Source: CAD feature listing. Evaluate the final solid. Frame: model axes, mm. A direction names the side the tool comes from. Round coordinates to 2 decimals unless told otherwise and drop trailing zeros. Order: outer loops, then holes, each group sorted by start corner. A loop starts at its lowest first (then second) coordinate and runs counter-clockwise, first axis right, second up. Notation, with made-up numbers: M 16.25,-26.5 L 46.25,-26.5 A30 ccw 46.25,-3.5 Z; hole C 10,81 d8. An arc over 180 degrees is marked long. Use one line per item in the form item = value. Start each with the question number.
Q1. Reachability of faces 1 (the flat face through (45, 10, 0.745)), 2 (the flat face through (45, -10, -0.745)), 3 (the cylindrical face through (4.7, 11.51, 3.62)) from +Z, -Z, +X, -X, +Y, -Y: full face, straight path, thin tool, end or side. Return the list, or none.
Q2. Section C-C (y = 0). Return the cut outline in (x, z) (3 decimals).
Q3. Pull-direction query (Y, two-part tool) for faces 4 (the cylindrical face through (50.978, 0.059, 3.174)), 5 (the cylindrical face through (36.13, 16.1, 5.07)), 6 (the flat face through (9.525, 11, -7)); classes: pulls with the +Y half, pulls with the -Y half, needs draft (parallel to the pull), parting line crosses it, or undercut.
Q4. Section A-A (x = 51). Return the cut outline in (y, z) (3 decimals), plus the area to 3 significant figures.
Q5. Material intervals for probe 1 along Z at (x, y) = (0.5, -0.5); probe 2 along Z at (x, y) = (51.5, 9), sorted ascending.
Q6. Section D-D (x = 16). Return the cut outline in (y, z).
Q7. Section B-B (z = 4.5). Return the cut outline in (x, y) (3 decimals).
Q8. Contact query for flat-ended pins moving along their axis: pin 1 (11 mm diameter, centred on x = 49.5, y = 7, fed in from -Z); pin 2 (6 mm diameter, centred on x = 5, z = -6, fed in from -Y); pin 3 (4 mm diameter, centred on x = 11, y = -2.5, fed in from -Z). Output: stop coordinate, or through.
from build123d import *

# Parameters (mm, degrees)
F0_R     = 12.065
F1_DEPTH = 9.525
F2_R     = 16.8783
F2_R_2   = 12.065
F3_DEPTH = 53.975
F4_R     = 12.7
F4_R_2   = 12.065
F5_DEPTH = 38.1
F6_R     = 3.175
F7_DEPTH = 25.4
F9_DEPTH = 38.1


with BuildPart() as f1:
    # F0 (on Right) → F1 (new body)
    with BuildSketch(Plane.YZ):
        Circle(F0_R)
    extrude(amount=F1_DEPTH)

    # F2 (on face) → F3 (join)
    with BuildSketch(Plane.YZ.offset(9.525)):
        Circle(F2_R)
        Circle(F2_R_2, mode=Mode.SUBTRACT)
        Circle(F2_R_2)
    extrude(amount=F3_DEPTH)

    # F4 (on face) → F5 (join)
    with BuildSketch(Plane(origin=(0, 0, 0), x_dir=(0, -1, 0), z_dir=(-1, 0, 0))):
        Circle(F4_R)
        Circle(F4_R_2, mode=Mode.SUBTRACT)
        Circle(F4_R_2)
    extrude(amount=F5_DEPTH)

    # F6 (on face) → F7 (cut)
    with BuildSketch(Plane.YZ.offset(63.5)):
        Circle(F6_R)
    extrude(amount=-F7_DEPTH, mode=Mode.SUBTRACT)

    # F8 (on face) → F9 (cut)
    with BuildSketch(Plane.YZ.offset(63.5)):
        with BuildLine():
            ThreePointArc((-16.8618667917, 0.7446201635), (-16.8783, 0), (-16.8618667917, -0.7446201635))
            Line((-16.8618667917, -0.7446201635), (-3.086448738, -0.7446201635))
            ThreePointArc((-3.086448738, -0.7446201635), (-3.175, 0), (-3.086448738, 0.7446201635))
            Line((-3.086448738, 0.7446201635), (-16.8618667917, 0.7446201635))
        make_face()
        with BuildLine():
            Line((3.086448738, -0.7446201635), (16.8618667917, -0.7446201635))
            ThreePointArc((16.8618667917, -0.7446201635), (16.8741911978, -0.3724007378), (16.8783, 0))
            ThreePointArc((16.8783, 0), (16.8741911978, 0.3724007378), (16.8618667917, 0.7446201635))
            Line((16.8618667917, 0.7446201635), (3.086448738, 0.7446201635))
            ThreePointArc((3.086448738, 0.7446201635), (3.1527844632, 0.3749334987), (3.175, 0))
            ThreePointArc((3.175, 0), (3.1527844632, -0.3749334987), (3.086448738, -0.7446201635))
        make_face()
    extrude(amount=-F9_DEPTH, mode=Mode.SUBTRACT)


solid = f1.part
Results list:
q1.face_1 = +X, +Y
q1.face_2 = +X, -Y
q1.face_3 = none
q2.outline = M -38.1,-12.7 L 0,-12.7 L 0,-12.065 L 9.525,-12.065 L 9.525,-16.878 L 63.5,-16.878 L 63.5,-3.175 L 38.1,-3.175 L 38.1,3.175 L 63.5,3.175 L 63.5,16.878 L 9.525,16.878 L 9.525,12.065 L 0,12.065 L 0,12.7 L -38.1,12.7 Z
q3.face_4 = undercut
q3.face_5 = parting line crosses it
q3.face_6 = needs draft
q4.outline = M -16.862,-0.745 A16.878 ccw 16.862,-0.745 L 3.086,-0.745 A3.175 cw -3.086,-0.745 Z; M -16.862,0.745 L -3.086,0.745 A3.175 cw 3.086,0.745 L 16.862,0.745 A16.878 ccw Z
q4.area = 822 mm2
q5.probe_1 = -12.05 to 12.05
q5.probe_2 = -14.28 to -0.74, 0.74 to 14.28
q6.outline = C 0,0 d33.76
q7.outline = M -38.1,-11.876 L 0,-11.876 L 0,-11.194 L 9.525,-11.194 L 9.525,-16.267 L 63.5,-16.267 L 63.5,16.267 L 9.525,16.267 L 9.525,11.194 L 0,11.194 L 0,11.876 L -38.1,11.876 Z
q8.pin_1 = -16.81
q8.pin_2 = -11.69
q8.pin_3 = -16.87
